Design review of the part shown in the three views and the two pictorial views. Dimensions are in mm from the part's minimum x, y and z. A direction names the side the tool comes from. Coordinates: 2 decimals unless noted, no trailing zeros. Loops run counter-clockwise (first coordinate to the right, second up) from the corner with the lowest first, then second, coordinate; pieces in that order, holes last. Notation, with made-up numbers: M 86,17 L 127,17 A26 ccw 127,31 Z; hole C -36,60.25 d4. An arc over 180 degrees is marked long. Answer as a JSON object with one key per item and string values. Group by question number.
Item 1: Wall thickness on L1, parallel to Y at x = 8, z = 5.3; L2, parallel to X at y = 7.25, z = 3.25 (1 decimal); L3, parallel to Z at x = 9, y = 6: over which ranges is each line inside the solid? List them lowest first. Write a range as from..to.
Item 2: Add section A-A (z = 3.5). State the section outline as (x, y) points.
Item 3: Insertion check: pin 1 (1 mm diameter, centred on x = 7, z = 4, fed in from -Y); pin 2 (2 mm diameter, centred on y = 4, z = 5, fed in from +X); pin 3 (3 mm diameter, centred on y = 2.5, z = 5.5, fed in from -X). Each pin has a flat end and moves straight along its axis. Give the tip position at first contact, or say it passes through.
Item 4: Tool access review of the marked faces 5 and 6: name each direction out of +Z, -Z, +X, -X, +Y, -Y from which nothing blocks a thin tool from reaching the whole face with its end or side.
Item 5: Mouldability with a two-part tool opening along Y and no side actions: class the marked faces 1, 2, 3 and 4 as +Y half, -Y half, draft (parallel to the pull), parting line (faces both ways), or undercut.
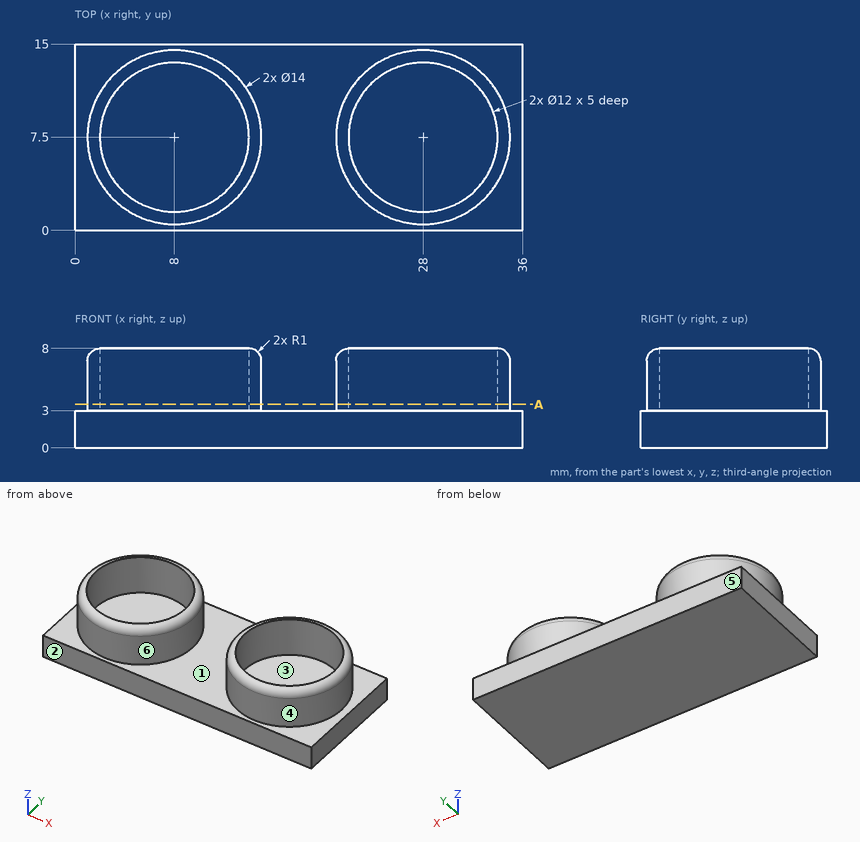
From the geometry:
{
 "1": {"L1": "y = 0.5..1.5, 13.5..14.5", "L2": "x = 1..2, 14..15, 21..22, 34..35", "L3": "z = 0..3"},
 "2": {"outline": "C 8,7.5 d14; C 28,7.5 d14; hole C 8,7.5 d12; hole C 28,7.5 d12"},
 "3": {"pin 1": "stops at y = 0.52", "pin 2": "stops at x = 34.54", "pin 3": "stops at x = 1.94"},
 "4": {"face 5": "+Z, -Z, +X, -X, +Y", "face 6": "+Z"},
 "5": {"face 1": "draft", "face 2": "-Y half", "face 3": "undercut", "face 4": "parting line"}
}
